Design review of the part shown in the three views and the two pictorial views. Dimensions are in mm from the part's minimum x, y and z. A direction names the side the tool comes from. Round coordinates to 2 decimals unless told otherwise and drop trailing zeros. Write each loop counter-clockwise with the first axis right and the second up, starting at its lowest first coordinate (ties: lowest second). Pieces come first, ordered by that corner, then holes. Notation, with made-up numbers: (58.5, 81.5) - (77.5, 81.5) arc R12 cw to (77.5, 96.5) - close; hole circle Ø6 at (-10.5, -36). An arc over 180 degrees is marked (long way). One line per item, written item: value. Start each with the question number.
Q1. Add section A-A on x = 15. Write out the cut boundary in (y, z), and give its area (3 significant figures).
Q2. Mouldability with a two-part tool opening along X and no side actions: class the marked faces 3, 4 and 5 as +X half, -X half, draft (parallel to the pull), parting line (faces both ways), or undercut.
Q3. Clearance check with flat-ended pins moving along their axes: pin 1 Ø4 at (x, y) = (10, 6.5) entering from +Z; pin 2 Ø1.5 at (x, y) = (25.5, 4.5) entering from +Z; pin 3 Ø1.2 at (y, z) = (6.5, 6) entering from +X; pin 4 Ø6 at (x, z) = (21, 15) entering from +Y. State where each tip first meets the part, or that it passes through.
Q4. Add section C-C on z = 15. Write out the cut boundary in (x, y).
Q5. Tool access review of the marked faces 1 and 2: name each direction out of +Z, -Z, +X, -X, +Y, -Y from which nothing blocks a thin tool from reaching the whole face with its end or side.
Q6. Add section B-B on y = 8.25. Write out the cut boundary in (x, z).
Q7. For probe 1 along X at (y, z) = (6.75, 15.25); probe 2 along X at (y, z) = (0.75, 19.25); probe 3 along Z at (x, y) = (21.5, 7.5) (1 decimal), list the stretches that pass through material, from the lowest coordinate up.
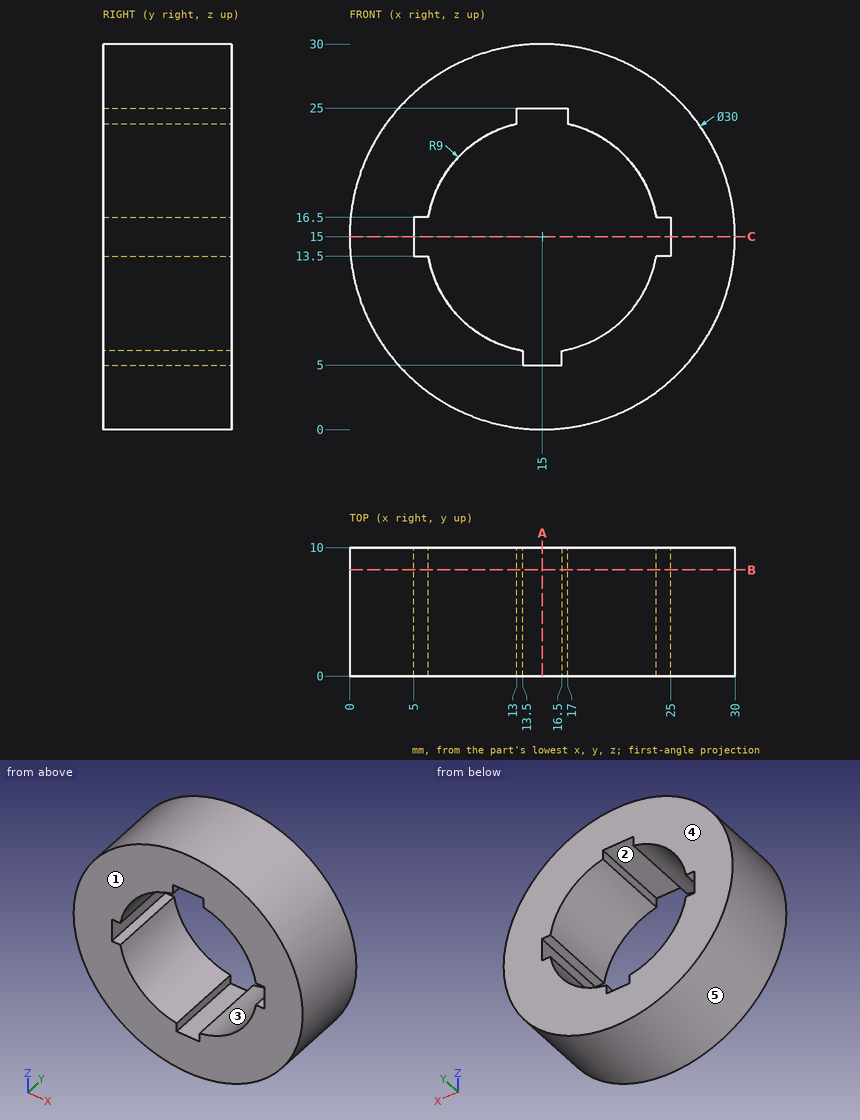
Result set:
1. outline: (0, 0) - (10, 0) - (10, 5) - (0, 5) - close; (0, 25) - (10, 25) - (10, 30) - (0, 30) - close
1. area: 100 mm^2
2. face 3: undercut
2. face 4: draft
2. face 5: parting line
3. pin 1: stops at z = 29.7
3. pin 2: stops at z = 26.4
3. pin 3: stops at x = 27.43
3. pin 4: passes through
4. outline: (0, 0) - (5, 0) - (5, 10) - (0, 10) - close; (25, 0) - (30, 0) - (30, 10) - (25, 10) - close
5. face 1: +Z, -Z, +X, -X, -Y
5. face 2: +Y, -Y
6. outline: circle Ø30 at (15, 15); hole (5, 13.5) - (6.13, 13.5) arc R9 ccw to (13.5, 6.13) - (13.5, 5) - (16.5, 5) - (16.5, 6.13) arc R9 ccw to (23.87, 13.5) - (25, 13.5) - (25, 16.5) - (23.87, 16.5) arc R9 ccw to (17, 23.77) - (17, 25) - (13, 25) - (13, 23.77) arc R9 ccw to (6.13, 16.5) - (5, 16.5) - close
7. probe 1: x = 0 to 5, 25 to 30
7. probe 2: x = 0.61 to 7.07, 22.93 to 29.39
7. probe 3: z = 1.5 to 8.8, 21.2 to 28.5
